Source: CAD feature listing. Evaluate the final solid. Frame: model axes, mm. A direction names the side the tool comes from. Round coordinates to 2 decimals unless told otherwise and drop trailing zeros. Loops run counter-clockwise (first coordinate to the right, second up) from the corner with the lowest first, then second, coordinate; pieces in that order, holes last. Notation, with made-up numbers: M 10,-21 L 52,-21 A11 cw 52,-13 Z; hole C 67,-21 d5. An arc over 180 degrees is marked long. Answer as a JSON object with one key per item and string values.
from build123d import *

# Parameters (mm, degrees)
SKETCH1_R           = 1.25
BOSS_EXTRUDE1_DEPTH = 2
BOSS_EXTRUDE2_DEPTH = 4
FILLET1_R           = 2
SKETCH3_W           = 2.4
SKETCH3_H           = 3.015421202
CUT_EXTRUDE1_DEPTH  = 4


with BuildPart() as part:
    # Sketch1 → Boss-Extrude1 (new body)
    with BuildSketch(Plane.XY):
        with BuildLine():
            Line((-7.5, -1.25), (-3, -1.25))
            ThreePointArc((-3, -1.25), (0, 3.25), (3, -1.25))
            Line((3, -1.25), (7.5, -1.25))
            ThreePointArc((7.5, -1.25), (10, -3.75), (7.5, -6.25))
            Line((7.5, -6.25), (-7.5, -6.25))
            ThreePointArc((-7.5, -6.25), (-10, -3.75), (-7.5, -1.25))
        make_face()
        Circle(SKETCH1_R, mode=Mode.SUBTRACT)
    extrude(amount=BOSS_EXTRUDE1_DEPTH)

    # Sketch2 → Boss-Extrude2 (add)
    with BuildSketch(Plane.XY.offset(2)):
        with BuildLine():
            Line((-8, -6.199489743), (-8, -1.300510257))
            ThreePointArc((-8, -1.300510257), (-10, -3.75), (-8, -6.199489743))
        make_face()
        with BuildLine():
            ThreePointArc((3, -1.703672504), (0, -3.45), (-3, -1.703672504))
            Line((-3, -1.703672504), (-3, -6.25))
            Line((-3, -6.25), (3, -6.25))
            Line((3, -6.25), (3, -1.703672504))
        make_face()
        with BuildLine():
            ThreePointArc((8, -6.199489743), (10, -3.75), (8, -1.300510257))
            Line((8, -1.300510257), (8, -6.199489743))
        make_face()
    extrude(amount=BOSS_EXTRUDE2_DEPTH)

    # Fillet1
    fillet1_edges = [part.edges().sort_by_distance(p)[0] for p in [
        (3, -1.25, 1),
        (-3, -1.25, 1),
    ]]
    fillet(fillet1_edges, radius=FILLET1_R)

    # Sketch3 → Cut-Extrude1 (cut)
    with BuildSketch(Plane.XY.offset(6)):
        with Locations((0, -4.742289399)):
            Rectangle(SKETCH3_W, SKETCH3_H)
    extrude(amount=-CUT_EXTRUDE1_DEPTH, mode=Mode.SUBTRACT)


solid = part.part
Item 1: Section C-C on y = 0. Return the cut outline in (x, z).
Answer sheet:
{"outline": "M -3.34,0 L -1.25,0 L -1.25,2 L -3.34,2 Z; M 1.25,0 L 3.34,0 L 3.34,2 L 1.25,2 Z"}
Item 2: Line query: probe 1 along X at (y, z) = (-4.5, 3); probe 2 along Z at (x, y) = (-1.5, 1.5); probe 3 along X at (y, z) = (-4.75, 3.85). Output: solid intervals per line, ascending. Write a range as from..to.
Answer sheet:
{"probe 1": "x = -9.88..-8, -3..-1.2, 1.2..3, 8..9.88", "probe 2": "z = 0..2", "probe 3": "x = -9.79..-8, -3..-1.2, 1.2..3, 8..9.79"}
Item 3: Section D-D on y = -3.75. Return the cut outline in (x, z).
Answer sheet:
{"outline": "M -10,0 L 10,0 L 10,6 L 8,6 L 8,2 L 3,2 L 3,6 L 1.2,6 L 1.2,2 L -1.2,2 L -1.2,6 L -3,6 L -3,2 L -8,2 L -8,6 L -10,6 Z"}
Item 4: Section B-B on z = 0.4. Return the cut outline in (x, y).
Answer sheet:
{"outline": "M -7.5,-6.25 L 7.5,-6.25 A2.5 ccw 7.5,-1.25 L 5.2,-1.25 A2 cw 3.22,0.46 A3.25 ccw -3.22,0.46 A2 cw -5.2,-1.25 L -7.5,-1.25 A2.5 ccw Z; hole C 0,0 d2.5"}
Item 5: Contact query for flat-ended pins moving along their axis: pin 1 Ø0.9 at (y, z) = (-4.5, 3) entering from +X; pin 2 Ø0.6 at (x, z) = (-7, 1) entering from +Y; pin 3 Ø1.5 at (y, z) = (2, 2) entering from -X. Output: stop coordinate, or through.
Answer sheet:
{"pin 1": "stops at x = 9.98", "pin 2": "stops at y = -1.25", "pin 3": "stops at x = -3"}
Item 6: Section A-A on x = 0. Return the cut outline in (y, z).
Answer sheet:
{"outline": "M -6.25,0 L -1.25,0 L -1.25,2 L -6.25,2 Z; M 1.25,0 L 3.25,0 L 3.25,2 L 1.25,2 Z"}
Item 7: Access query for faces 4 (the flat face through (8, -4, 4)), 5 (the flat face through (-9, -4, 6)), 6 (the cylindrical face through (2.248, -2.617, 3.972)), 7 (the cylindrical face through (-3.902, -0.775, 1.014)), 8 (the flat face through (6, -1.25, 1)). Directions: +Z, -Z, +X, -X, +Y, -Y. A direction counts if a zero-diameter tool reaches every point of the face in a straight line with its end or side. Return the directions, or none.
Answer sheet:
{"face 4": "+Z, +Y, -Y", "face 5": "+Z, +X, -X, +Y, -Y", "face 6": "+Z, +Y", "face 7": "+Z, -Z, -X, +Y", "face 8": "+Z, -Z, +X, +Y"}
Item 8: Pull-direction query (X, two-part tool) for faces 1 (the flat face through (-2, -4, 6)), 2 (the cylindrical face through (3.872, -0.749, 1.014)), 3 (the flat face through (3, -4, 4)); classes: pulls with the +X half, pulls with the -X half, needs draft (parallel to the pull), parting line crosses it, or undercut.
Answer sheet:
{"face 1": "needs draft", "face 2": "pulls with the +X half", "face 3": "undercut"}
